Verification items for the finished model (mm, model axes). A direction names the side the tool comes from. Coordinates: 2 decimals unless noted, no trailing zeros. Loops run counter-clockwise (first coordinate to the right, second up) from the corner with the lowest first, then second, coordinate; pieces in that order, holes last. Notation, with made-up numbers: (57, -28) -> (70, -28) arc R26 ccw to (70, -10) -> close; hole circle Ø4 at (36.5, -33.5). An arc over 180 degrees is marked (long way). Answer as a JSON object with one key per item and string values. Group by question number.
Q1. Set-up check for faces 5 (the flat face through (3, -139.75, -11)), 6 (the flat face through (-4, 2, -1)), 7 (the flat face through (-3, 140.75, -11)), 8 (the flat face through (-253, -1, -11)): record each of +Z, -Z, +X, -X, +Y, -Y from which the full face is reachable in a straight line by a thin tool's end or side.
Q2. Cross-section at B-B on y = -60.75. Record the boundary of the cut face in (x, z), and give its area (3 significant figures).
Q3. Release check for a two-part mould opening along Y. For faces 1 (the flat face through (-3, 139.75, -11)), 2 (the flat face through (-4, 2, 0)), 3 (the flat face through (3, -140.75, -11)), 4 (the cylindrical face through (202.615, -51.739, -0.493)) record: released by +Y, released by -Y, zero draft, split by the parting line, or undercut.
Q4. Gauge pin test, flat ends, axial feed: pin 1 Ø1.2 at (x, z) = (253, -6) entering from +Y; pin 2 Ø1.5 at (x, y) = (83, 16) entering from -Z; pin 3 Ø0.8 at (y, z) = (140, -14.5) entering from -X. Record the tip position at first contact, or that the pin passes through.
Q5. Scan lines: L1, parallel to X at y = 130.75, z = -0.7; L2, parallel to X at y = 140.4, z = -10; L3, parallel to Y at x = 244, z = -0.45. Record each from-to range of solid material in increasing order.
Q6. Cross-section at A-A on x = 174. Record the boundary of the cut face in (y, z), and give its area (3 significant figures).
Q7. Cross-section at C-C on z = -9.25. Record the boundary of the cut face in (x, y).
Q8. Cross-section at D-D on y = 42.5. Record the boundary of the cut face in (x, z).
```python
from build123d import *

# Parameters (mm, degrees)
SKETCH_1_W                        = 508
SKETCH_1_H                        = 281.5
SKETCH_1_R                        = 3
SKETCH_1_R_2                      = 30
SKETCH_1_W_2                      = 94
SKETCH_1_H_2                      = 46
SM_BASE_FLANGE_1_DEPTH            = 1
SM_EDGE_FLANGE_1_STRIP_W          = 5
SM_EDGE_FLANGE_1_STRIP_H          = 1
SM_EDGE_FLANGE_1_STRIP_CUT_DEPTH  = 408
SM_EDGE_FLANGE_1_RELIEF_W         = 6
SM_EDGE_FLANGE_1_RELIEF_H         = 1
SM_EDGE_FLANGE_1_RELIEF_CUT_DEPTH = 1
SM_EDGE_FLANGE_1_DEPTH            = 408
SM_EDGE_FLANGE_2_STRIP_W          = 5
SM_EDGE_FLANGE_2_STRIP_H          = 1
SM_EDGE_FLANGE_2_STRIP_CUT_DEPTH  = 181.5
SM_EDGE_FLANGE_2_RELIEF_W         = 6
SM_EDGE_FLANGE_2_RELIEF_H         = 1
SM_EDGE_FLANGE_2_RELIEF_CUT_DEPTH = 1
SM_EDGE_FLANGE_2_DEPTH            = 181.5
SM_EDGE_FLANGE_3_STRIP_W          = 5
SM_EDGE_FLANGE_3_STRIP_H          = 1
SM_EDGE_FLANGE_3_STRIP_CUT_DEPTH  = 408
SM_EDGE_FLANGE_3_RELIEF_W         = 6
SM_EDGE_FLANGE_3_RELIEF_H         = 1
SM_EDGE_FLANGE_3_RELIEF_CUT_DEPTH = 1
SM_EDGE_FLANGE_3_DEPTH            = 408
SM_EDGE_FLANGE_4_STRIP_W          = 5
SM_EDGE_FLANGE_4_STRIP_H          = 1
SM_EDGE_FLANGE_4_STRIP_CUT_DEPTH  = 181.5
SM_EDGE_FLANGE_4_RELIEF_W         = 6
SM_EDGE_FLANGE_4_RELIEF_H         = 1
SM_EDGE_FLANGE_4_RELIEF_CUT_DEPTH = 1
SM_EDGE_FLANGE_4_DEPTH            = 181.5
SKETCH_32_R                       = 4
CUT_EXTRUDE_1_DEPTH               = 379.940958462


# Sheet-metal steps are written as plain solids
with BuildPart() as part:
    # 基体-法兰1: sheet metal written as solids
    # Sketch 1 → 基体-法兰1 (new body)
    with BuildSketch(Plane.XY):
        Rectangle(SKETCH_1_W, SKETCH_1_H)
        with Locations((-244, 130.75)):
            Circle(SKETCH_1_R, mode=Mode.SUBTRACT)
        with Locations((-244, -130.75)):
            Circle(SKETCH_1_R, mode=Mode.SUBTRACT)
        with Locations((244, 130.75)):
            Circle(SKETCH_1_R, mode=Mode.SUBTRACT)
        with Locations((244, -130.75)):
            Circle(SKETCH_1_R, mode=Mode.SUBTRACT)
        with Locations((174, -60.75)):
            Circle(SKETCH_1_R_2, mode=Mode.SUBTRACT)
        with Locations((95.5, 99.75)):
            Rectangle(SKETCH_1_W_2, SKETCH_1_H_2, mode=Mode.SUBTRACT)
    extrude(amount=-SM_BASE_FLANGE_1_DEPTH)

    # 边线-法兰1: sheet metal written as solids
    # 边线-法兰1 strip (on a plane across the edge) → 边线-法兰1 strip cut (cut)
    with BuildSketch(Plane(origin=(-204, 140.75, -1), x_dir=(0, -1, 0), z_dir=(1, 0, 0))):
        with Locations((-1, -0.5)):
            Rectangle(SM_EDGE_FLANGE_1_STRIP_W, SM_EDGE_FLANGE_1_STRIP_H)
    extrude(amount=SM_EDGE_FLANGE_1_STRIP_CUT_DEPTH, mode=Mode.SUBTRACT)

    # 边线-法兰1 relief (on the sheet) → 边线-法兰1 relief cut (cut)
    with BuildSketch(Plane(origin=(-204, 139.25, -1), x_dir=(0, -1, 0), z_dir=(0, 0, -1))):
        with Locations((-2, 0.5)):
            Rectangle(SM_EDGE_FLANGE_1_RELIEF_W, SM_EDGE_FLANGE_1_RELIEF_H)
        with Locations((-2, -408.5)):
            Rectangle(SM_EDGE_FLANGE_1_RELIEF_W, SM_EDGE_FLANGE_1_RELIEF_H)
    extrude(amount=-SM_EDGE_FLANGE_1_RELIEF_CUT_DEPTH, mode=Mode.SUBTRACT)

    # 边线-法兰1 section (on a plane across the edge) → 边线-法兰1 (add)
    with BuildSketch(Plane(origin=(-204, 140.75, -1), x_dir=(0, -1, 0), z_dir=(1, 0, 0))):
        with BuildLine():
            Line((0, 0.5), (0, 19))
            Line((0, 19), (1, 19))
            Line((1, 19), (1, 0.5))
            ThreePointArc((1, 0.5), (1.146446609, 0.146446609), (1.5, 0))
            Line((1.5, 0), (1.5, -1))
            ThreePointArc((1.5, -1), (0.439339828, -0.560660172), (0, 0.5))
        make_face()
    extrude(amount=SM_EDGE_FLANGE_1_DEPTH)

    # 边线-法兰2: sheet metal written as solids
    # 边线-法兰2 strip (on a plane across the edge) → 边线-法兰2 strip cut (cut)
    with BuildSketch(Plane(origin=(-254, -90.75, -1), x_dir=(1, 0, 0), z_dir=(0, 1, 0))):
        with Locations((-1, -0.5)):
            Rectangle(SM_EDGE_FLANGE_2_STRIP_W, SM_EDGE_FLANGE_2_STRIP_H)
    extrude(amount=SM_EDGE_FLANGE_2_STRIP_CUT_DEPTH, mode=Mode.SUBTRACT)

    # 边线-法兰2 relief (on the sheet) → 边线-法兰2 relief cut (cut)
    with BuildSketch(Plane(origin=(-252.5, -90.75, -1), x_dir=(1, 0, 0), z_dir=(0, 0, -1))):
        with Locations((-2, 0.5)):
            Rectangle(SM_EDGE_FLANGE_2_RELIEF_W, SM_EDGE_FLANGE_2_RELIEF_H)
        with Locations((-2, -182)):
            Rectangle(SM_EDGE_FLANGE_2_RELIEF_W, SM_EDGE_FLANGE_2_RELIEF_H)
    extrude(amount=-SM_EDGE_FLANGE_2_RELIEF_CUT_DEPTH, mode=Mode.SUBTRACT)

    # 边线-法兰2 section (on a plane across the edge) → 边线-法兰2 (add)
    with BuildSketch(Plane(origin=(-254, -90.75, -1), x_dir=(1, 0, 0), z_dir=(0, 1, 0))):
        with BuildLine():
            Line((0, 0.5), (0, 19))
            Line((0, 19), (1, 19))
            Line((1, 19), (1, 0.5))
            ThreePointArc((1, 0.5), (1.146446609, 0.146446609), (1.5, 0))
            Line((1.5, 0), (1.5, -1))
            ThreePointArc((1.5, -1), (0.439339828, -0.560660172), (0, 0.5))
        make_face()
    extrude(amount=SM_EDGE_FLANGE_2_DEPTH)

    # 边线-法兰3: sheet metal written as solids
    # 边线-法兰3 strip (on a plane across the edge) → 边线-法兰3 strip cut (cut)
    with BuildSketch(Plane(origin=(204, -140.75, -1), x_dir=(0, 1, 0), z_dir=(-1, 0, 0))):
        with Locations((-1, -0.5)):
            Rectangle(SM_EDGE_FLANGE_3_STRIP_W, SM_EDGE_FLANGE_3_STRIP_H)
    extrude(amount=SM_EDGE_FLANGE_3_STRIP_CUT_DEPTH, mode=Mode.SUBTRACT)

    # 边线-法兰3 relief (on the sheet) → 边线-法兰3 relief cut (cut)
    with BuildSketch(Plane(origin=(204, -139.25, -1), x_dir=(0, 1, 0), z_dir=(0, 0, -1))):
        with Locations((-2, 0.5)):
            Rectangle(SM_EDGE_FLANGE_3_RELIEF_W, SM_EDGE_FLANGE_3_RELIEF_H)
        with Locations((-2, -408.5)):
            Rectangle(SM_EDGE_FLANGE_3_RELIEF_W, SM_EDGE_FLANGE_3_RELIEF_H)
    extrude(amount=-SM_EDGE_FLANGE_3_RELIEF_CUT_DEPTH, mode=Mode.SUBTRACT)

    # 边线-法兰3 section (on a plane across the edge) → 边线-法兰3 (add)
    with BuildSketch(Plane(origin=(204, -140.75, -1), x_dir=(0, 1, 0), z_dir=(-1, 0, 0))):
        with BuildLine():
            Line((0, 0.5), (0, 19))
            Line((0, 19), (1, 19))
            Line((1, 19), (1, 0.5))
            ThreePointArc((1, 0.5), (1.146446609, 0.146446609), (1.5, 0))
            Line((1.5, 0), (1.5, -1))
            ThreePointArc((1.5, -1), (0.439339828, -0.560660172), (0, 0.5))
        make_face()
    extrude(amount=SM_EDGE_FLANGE_3_DEPTH)

    # 边线-法兰4: sheet metal written as solids
    # 边线-法兰4 strip (on a plane across the edge) → 边线-法兰4 strip cut (cut)
    with BuildSketch(Plane(origin=(254, 90.75, -1), x_dir=(-1, 0, 0), z_dir=(0, -1, 0))):
        with Locations((-1, -0.5)):
            Rectangle(SM_EDGE_FLANGE_4_STRIP_W, SM_EDGE_FLANGE_4_STRIP_H)
    extrude(amount=SM_EDGE_FLANGE_4_STRIP_CUT_DEPTH, mode=Mode.SUBTRACT)

    # 边线-法兰4 relief (on the sheet) → 边线-法兰4 relief cut (cut)
    with BuildSketch(Plane(origin=(252.5, 90.75, -1), x_dir=(-1, 0, 0), z_dir=(0, 0, -1))):
        with Locations((-2, 0.5)):
            Rectangle(SM_EDGE_FLANGE_4_RELIEF_W, SM_EDGE_FLANGE_4_RELIEF_H)
        with Locations((-2, -182)):
            Rectangle(SM_EDGE_FLANGE_4_RELIEF_W, SM_EDGE_FLANGE_4_RELIEF_H)
    extrude(amount=-SM_EDGE_FLANGE_4_RELIEF_CUT_DEPTH, mode=Mode.SUBTRACT)

    # 边线-法兰4 section (on a plane across the edge) → 边线-法兰4 (add)
    with BuildSketch(Plane(origin=(254, 90.75, -1), x_dir=(-1, 0, 0), z_dir=(0, -1, 0))):
        with BuildLine():
            Line((0, 0.5), (0, 19))
            Line((0, 19), (1, 19))
            Line((1, 19), (1, 0.5))
            ThreePointArc((1, 0.5), (1.146446609, 0.146446609), (1.5, 0))
            Line((1.5, 0), (1.5, -1))
            ThreePointArc((1.5, -1), (0.439339828, -0.560660172), (0, 0.5))
        make_face()
    extrude(amount=SM_EDGE_FLANGE_4_DEPTH)

    # 草图32 → 切除-拉伸1 (cut, through all)
    with BuildSketch(Plane(origin=(0, 139.75, 0), x_dir=(-1, 0, 0), z_dir=(0, -1, 0))):
        with Locations(Location((-134.5, 10, 0), (0, 0, 90))):
            Circle(SKETCH_32_R)
        with Locations(Location((-56.5, 10, 0), (0, 0, 90))):
            Circle(SKETCH_32_R)
    extrude(amount=-CUT_EXTRUDE_1_DEPTH, mode=Mode.SUBTRACT)


solid = part.part
```
Computed values:
{
 "1": {"face 5": "-Z, +X, -X", "face 6": "-Z", "face 7": "+Z, -Z, +X, -X, +Y", "face 8": "-Z, +Y, -Y"},
 "2": {"outline": "(-254, -20) -> (-253, -20) -> (-253, -1.5) arc R0.5 cw to (-252.5, -1) -> (144, -1) -> (144, 0) -> (-252.5, 0) arc R1.5 ccw to (-254, -1.5) -> close; (204, -1) -> (252.5, -1) arc R0.5 cw to (253, -1.5) -> (253, -20) -> (254, -20) -> (254, -1.5) arc R1.5 ccw to (252.5, 0) -> (204, 0) -> close", "area": "485 mm²"},
 "3": {"face 1": "undercut", "face 2": "zero draft", "face 3": "released by -Y", "face 4": "undercut"},
 "4": {"pin 1": "stops at y = 90.75", "pin 2": "stops at z = -1", "pin 3": "stops at x = -204"},
 "5": {"L1": "x = -254 to -247, -241 to 241, 247 to 254", "L2": "x = -204 to 52.5, 60.5 to 130.5, 138.5 to 204", "L3": "y = -140.75 to -133.75, -127.75 to 127.75, 133.75 to 140.75"},
 "6": {"outline": "(-140.75, -20) -> (-139.75, -20) -> (-139.75, -1.5) arc R0.5 cw to (-139.25, -1) -> (-90.75, -1) -> (-90.75, 0) -> (-139.25, 0) arc R1.5 ccw to (-140.75, -1.5) -> close; (-30.75, -1) -> (139.25, -1) arc R0.5 cw to (139.75, -1.5) -> (139.75, -20) -> (140.75, -20) -> (140.75, -1.5) arc R1.5 ccw to (139.25, 0) -> (-30.75, 0) -> close", "area": "259 mm²"},
 "7": {"outline": "(-254, -90.75) -> (-253, -90.75) -> (-253, 90.75) -> (-254, 90.75) -> close; (-204, -140.75) -> (204, -140.75) -> (204, -139.75) -> (-204, -139.75) -> close; (-204, 139.75) -> (52.57, 139.75) -> (52.57, 140.75) -> (-204, 140.75) -> close; (60.43, 139.75) -> (130.57, 139.75) -> (130.57, 140.75) -> (60.43, 140.75) -> close; (138.43, 139.75) -> (204, 139.75) -> (204, 140.75) -> (138.43, 140.75) -> close; (253, -90.75) -> (254, -90.75) -> (254, 90.75) -> (253, 90.75) -> close"},
 "8": {"outline": "(-254, -20) -> (-253, -20) -> (-253, -1.5) arc R0.5 cw to (-252.5, -1) -> (252.5, -1) arc R0.5 cw to (253, -1.5) -> (253, -20) -> (254, -20) -> (254, -1.5) arc R1.5 ccw to (252.5, 0) -> (-252.5, 0) arc R1.5 ccw to (-254, -1.5) -> close"}
}
